Source: three-view drawing plus pictorial views. Frame: mm from the lowest corner of the part. Give positions to 0.01 mm unless a question says otherwise; leave off trailing zeros. Write each loop counter-clockwise with the first axis right and the second up, starting at its lowest first coordinate (ties: lowest second). Pieces come first, ordered by that corner, then holes. Notation, with made-up numbers: (24, -11) -> (40, -11) arc R17 ccw to (40, 22) -> close; hole circle Ø3 at (38, 89). An arc over 180 degrees is marked (long way). Answer in a Markdown table with one row per item. Add a question column.
Item 1: First-contact query: P1, Ø6, axis at y = 3.5, z = 16.5, coming from the +X side; P2, Ø2, axis at y = 6, z = 44.5, coming from the +X side (1 decimal); P3, Ø1, axis at y = 2, z = 20, coming from the +X side. Flat tips, straight axial feed; report the tip coordinate or a pass-through.
Item 2: Material intervals for probe 1 along Z at (x, y) = (27, 9.5); probe 2 along X at (y, z) = (9.5, 12.5) (1 decimal); probe 3 along X at (y, z) = (1.75, 36) (1 decimal), sorted ascending. Write a range as from..to.
Item 3: Draft query along X for the marked faces 1, 2 and 3. Return one class per face: +X half, -X half, draft (parallel to the pull), parting line (faces both ways), or undercut.
Item 4: Section query B-B on y = 4.5. Output: boundary loops of the cut face in (x, z) (1 decimal), plus the area to 3 significant figures.
Item 5: Section query D-D on y = 9.25. Output: boundary loops of the cut face in (x, z), plus the area to 3 significant figures.
Item 6: Section query A-A on z = 19. Output: boundary loops of the cut face in (x, y), plus the area to 3 significant figures.
Item 7: Section query C-C on x = 5. Output: boundary loops of the cut face in (y, z).
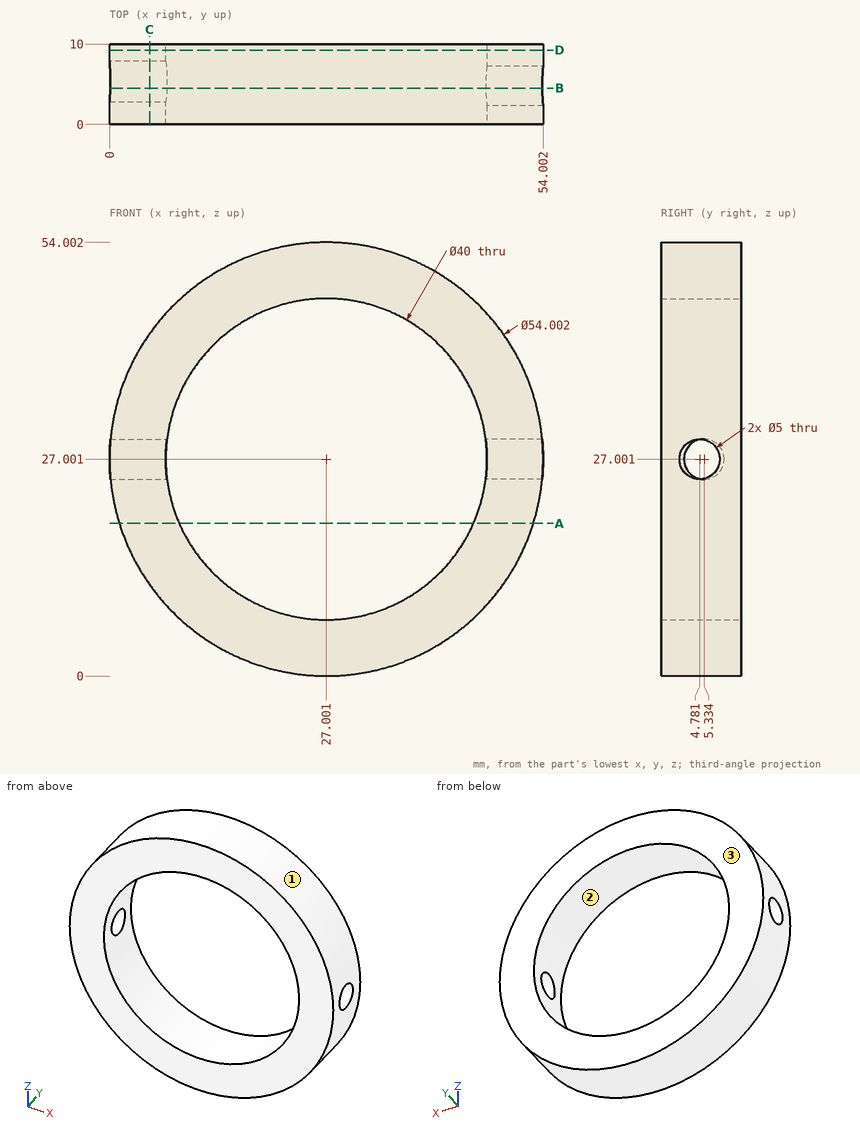
Findings below:
| question | item | result |
|---|---|---|
| 1 | P1 | stops at x = 52.94 |
| 1 | P2 | stops at x = 48.4 |
| 1 | P3 | stops at x = 53.21 |
| 2 | probe 1 | z = 0..7, 47..54 |
| 2 | probe 2 | x = 4.2..13.2, 40.8..49.8 |
| 2 | probe 3 | x = 1.5..9.1, 44.9..52.5 |
| 3 | face 1 | parting line |
| 3 | face 2 | undercut |
| 3 | face 3 | draft |
| 4 | outline | (0.1, 24.6) arc R27 ccw to (53.9, 24.5) -> (46.8, 24.5) arc R20 cw to (7.1, 24.6) -> close; (0.1, 29.4) -> (7.1, 29.4) arc R20 cw to (46.8, 29.5) -> (53.9, 29.5) arc R27 ccw to start |
| 4 | area | 966 mm^2 |
| 5 | outline | circle Ø54 at (27, 27); hole circle Ø40 at (27, 27) |
| 5 | area | 1,030 mm^2 |
| 6 | outline | (1.21, 0) -> (8.67, 0) -> (8.67, 10) -> (1.21, 10) -> close; (45.33, 0) -> (52.79, 0) -> (52.79, 10) -> (45.33, 10) -> close |
| 6 | area | 149 mm^2 |
| 7 | outline | (0, 11.35) -> (10, 11.35) -> (10, 42.65) -> (0, 42.65) -> close; hole circle Ø5 at (5.33, 27) |
